Work out the finished part from the listing and answer in its coordinate system (mm). A direction names the side the tool comes from. Give positions to 0.01 mm unless a question says otherwise; leave off trailing zeros. Loops run counter-clockwise (first coordinate to the right, second up) from the corner with the lowest first, then second, coordinate; pieces in that order, holes last. Notation, with made-up numbers: (-20, -3.5) - (6, -3.5) arc R17 ccw to (6, 20.5) - close; hole circle Ø7 at (23.5, 77). An arc over 180 degrees is marked (long way). One line per question, with ' | ' between items.
from build123d import *

# Parameters (mm, degrees)
SKETCH005_AS_DRAWN_R                                = 2.75
EXTRUDE_SKETCH005001_DEPTH                          = 90
EXTRUDE_SKETCH005001_ONTO_SKETCH005_ROLL_ANGLE      = 90
EXTRUDE_SKETCH005001_ONTO_SKETCH005_PLACEMENT_ANGLE = 180
CYLINDER_R                                          = 9
CYLINDER_DEPTH                                      = 80
CYLINDER001_R                                       = 9
CYLINDER001_DEPTH                                   = 80
CYLINDER001_ROLL_ANGLE                              = 90
CLONE005_PLACEMENT_ANGLE                            = 25


with BuildPart() as clone_of_sketch005_extrude001:
    # Sketch005 as drawn → Extrude_Sketch005001 (new)
    with BuildSketch(Plane.XY):
        with Locations((-90, 54)):
            Circle(SKETCH005_AS_DRAWN_R)
    extrude(amount=-EXTRUDE_SKETCH005001_DEPTH)


with BuildPart() as clone_of_sketch005_extrude001_1:
    # Extrude_Sketch005001 onto Sketch005 roll: moved
    add(clone_of_sketch005_extrude001.part.rotate(Axis((0, 0, 0), (1, 0, 0)), EXTRUDE_SKETCH005001_ONTO_SKETCH005_ROLL_ANGLE))


with BuildPart() as clone_of_sketch005_extrude001_2:
    # Extrude_Sketch005001 onto Sketch005 placement: moved
    add(clone_of_sketch005_extrude001_1.part.moved(Location((0, 111, 0))).rotate(Axis((0, 111, 0), (0, 0, 1)), EXTRUDE_SKETCH005001_ONTO_SKETCH005_PLACEMENT_ANGLE))


with BuildPart() as cilindro:
    # Cylinder → Cylinder (new body)
    with BuildSketch(Plane(origin=(76.968275, 45, 32), x_dir=(1, 0, 0), z_dir=(0, 0, 1))):
        Circle(CYLINDER_R)
    extrude(amount=CYLINDER_DEPTH)


with BuildPart() as clone_of_cilindro:
    # Clone003 base: copy of Cilindro
    add(cilindro.part)


with BuildPart() as clone_of_cilindro_1:
    # Clone003 placement: moved
    add(clone_of_cilindro.part.moved(Location((0, 50, 0))))


with BuildPart() as clone_of_cut003:
    # Cylinder001 → Cylinder001 (new body)
    with BuildSketch(Plane.XY):
        Circle(CYLINDER001_R)
    extrude(amount=CYLINDER001_DEPTH)


with BuildPart() as clone_of_cut003_1:
    # Cylinder001 roll: moved
    add(clone_of_cut003.part.rotate(Axis((0, 0, 0), (1, 0, 0)), CYLINDER001_ROLL_ANGLE))


with BuildPart() as clone_of_cut003_2:
    # Cylinder001 placement: moved
    add(clone_of_cut003_1.part.moved(Location((76.9683, 110, 112))))

    # Fusion: union Clone of Cilindro, Cilindro
    add(clone_of_cilindro_1.part)
    add(cilindro.part)


with BuildPart() as clone_of_cut003_3:
    # Fusion placement: moved
    add(clone_of_cut003_2.part.moved(Location((13.0317, 0, -18))))

    # Cut003: cut Clone of Sketch005_Extrude001
    add(clone_of_sketch005_extrude001_2.part, mode=Mode.SUBTRACT)


with BuildPart() as clone_of_cut003_4:
    # Clone005 placement: moved
    add(clone_of_cut003_3.part.moved(Location((31, 0, -33))).rotate(Axis((31, 0, -33), (0, -1, 0)), CLONE005_PLACEMENT_ANGLE))


solid = clone_of_cut003_4.part
1. Find section B-B on x = 89. State how many separate pieces and enclosed holes the cut face has, then the cut area to 3 significant figures.
Evaluation:
separate pieces: 4 | enclosed holes: 0 | area: 1,010 mm2
2. Find section D-D on y = 72. Write down the section's boundary in (x, z), then the cut area to 3 significant figures.
Evaluation:
outline: circle Ø18 at (72.84, 90.23) | area: 254 mm2
3. Find section A-A on y = 91. Write down the section's boundary in (x, z), then the cut area to 3 significant figures.
Evaluation:
outline: (67.23, 83.2) - (99.34, 14.32) - (113.96, 21.13) - (81.84, 90.01) arc R9 ccw (long way) to start; hole circle Ø5.5 at (89.75, 53.98) | area: 1,400 mm2
4. Flat-ended cylindrical pins translate along their axes: pin 1 (2 mm diameter, centred on x = 76.5, z = 70, fed in from +Y); pin 2 (10 mm diameter, centred on y = 55, z = 68, fed in from -X); pin 3 (4 mm diameter, centred on x = 75, z = 78, fed in from +Y). Find the tip coordinate at first contact, or state that the pin passes through.
Evaluation:
pin 1: y = 102.94 | pin 2: x = 74.33 | pin 3: y = 103.92
5. Determine the mould class of faces 1 (the flat face through (106.54, 45.13, 17.67)), 2 (the flat face through (73, 30, 90)), 3 (the cylindrical face through (87.02, 45.13, 53.62)) for opening direction Z: +Z half, -Z half, draft (parallel to the pull), parting line (faces both ways), or undercut.
Evaluation:
face 1: -Z half | face 2: draft | face 3: undercut
6. Consider L1, parallel to Y at x = 88, z = 44; L2, parallel to Y at x = 86, z = 76; L3, parallel to Z at x = 91, y = 96. Determine where each line is inside the solid, lowest interval first.
Evaluation:
L1: 38.12 to 51.88, 88.12 to 101.88 | L2: 38.21 to 51.79, 88.21 to 101.79 | L3: 30.12 to 51.53, 56.42 to 72.45
7. Which of the six approach directions +Z, -Z, +X, -X, +Y, -Y give full straight-line access (tool end or side, diameter ignored) to faces 4 (the cylindrical face through (68.01, 70.56, 97.82)), 5 (the flat face through (73, 110, 90))?
Evaluation:
face 4: none | face 5: +Z, -Z, +X, -X, +Y
